Source: three-view drawing plus pictorial views. Frame: mm from the lowest corner of the part. A direction names the side the tool comes from. Round coordinates to 2 decimals unless told otherwise and drop trailing zeros. Write each loop counter-clockwise with the first axis right and the second up, starting at its lowest first coordinate (ties: lowest second). Pieces come first, ordered by that corner, then holes. Notation, with made-up numbers: M 8,-33.75 L 55,-33.75 A30 cw 55,-11.75 Z; hole C 23.5,60.25 d2. An arc over 180 degrees is marked long. Answer in a Markdown table with one row per item.
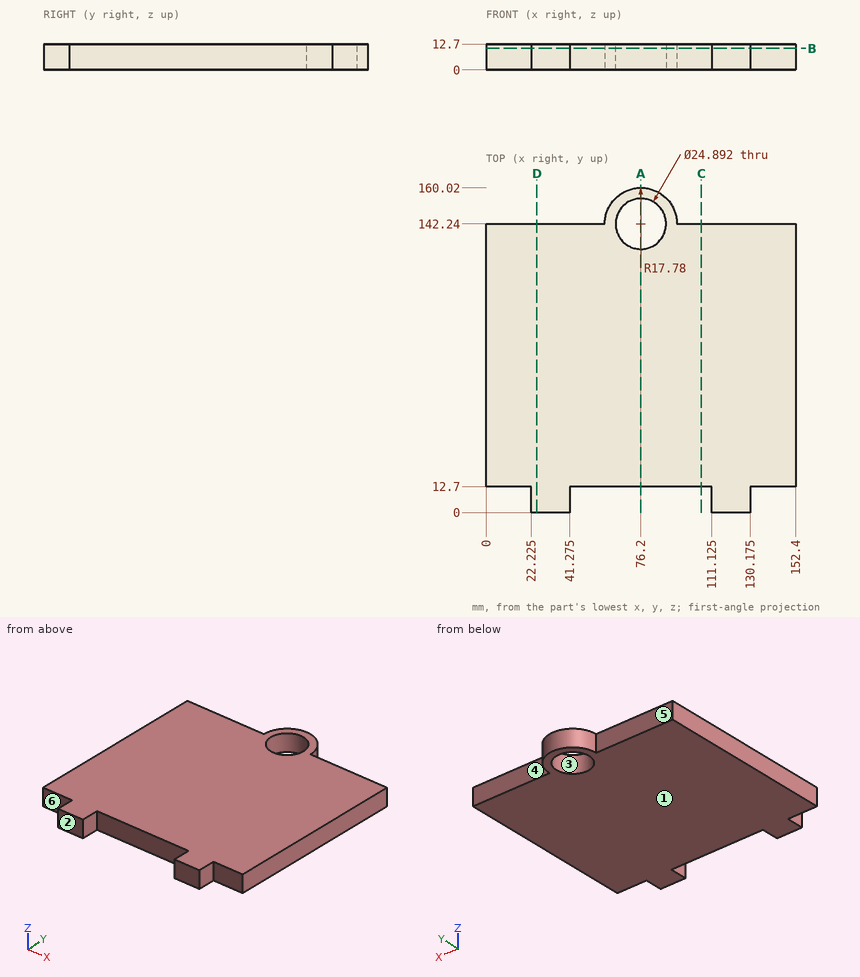
Q1. Section B-B (z = 10.5). Return loops of the section in (x, y) (3 decimals), and give its area (3 significant figures).
Solutions:
| item | result |
|---|---|
| outline | M 0,12.7 L 22.225,12.7 L 22.225,0 L 41.275,0 L 41.275,12.7 L 111.125,12.7 L 111.125,0 L 130.175,0 L 130.175,12.7 L 152.4,12.7 L 152.4,142.24 L 93.98,142.24 A17.78 ccw 58.42,142.24 L 0,142.24 Z; hole C 76.2,142.24 d24.892 |
| area | 20,200 mm2 |
Q2. Contact query for flat-ended pins moving along their axis: pin 1 Ø2 at (x, z) = (47, 6.5) entering from +Y; pin 2 Ø4 at (y, z) = (5, 4) entering from +X (3 decimals); pin 3 Ø6.5 at (y, z) = (8.5, 4.5) entering from -X (3 decimals). Output: stop coordinate, or through.
Solutions:
| item | result |
|---|---|
| pin 1 | stops at y = 142.24 |
| pin 2 | stops at x = 130.175 |
| pin 3 | stops at x = 22.225 |
Q3. Pull-direction query (Y, two-part tool) for the marked faces 1, 2 and 3; classes: pulls with the +Y half, pulls with the -Y half, needs draft (parallel to the pull), parting line crosses it, or undercut.
Solutions:
| item | result |
|---|---|
| face 1 | needs draft |
| face 2 | pulls with the -Y half |
| face 3 | undercut |
Q4. Access query for the marked faces 4, 5 and 6. Directions: +Z, -Z, +X, -X, +Y, -Y. A direction counts if a zero-diameter tool reaches every point of the face in a straight line with its end or side. Return the directions, or none.
Solutions:
| item | result |
|---|---|
| face 4 | +Z, -Z, +X, +Y |
| face 5 | +Z, -Z, -X, +Y |
| face 6 | +Z, -Z, -X, -Y |
Q5. Section D-D (x = 25). Return loops of the section in (y, z).
Solutions:
| item | result |
|---|---|
| outline | M 0,0 L 142.24,0 L 142.24,12.7 L 0,12.7 Z |
Q6. Section A-A (x = 76.2). Return loops of the section in (y, z), and give its area (3 significant figures).
Solutions:
| item | result |
|---|---|
| outline | M 12.7,0 L 129.79,0 L 129.79,12.7 L 12.7,12.7 Z; M 154.69,0 L 160.02,0 L 160.02,12.7 L 154.69,12.7 Z |
| area | 1,550 mm2 |
Q7. Material intervals for probe 1 along Y at (x, z) = (25, 9.25); probe 2 along Y at (x, z) = (108, 7); probe 3 along Y at (x, z) = (71, 5.5), sorted ascending.
Solutions:
| item | result |
|---|---|
| probe 1 | y = 0 to 142.24 |
| probe 2 | y = 12.7 to 142.24 |
| probe 3 | y = 12.7 to 130.93, 153.55 to 159.24 |
Q8. Section C-C (x = 106). Return loops of the section in (y, z), and give its area (3 significant figures).
Solutions:
| item | result |
|---|---|
| outline | M 12.7,0 L 142.24,0 L 142.24,12.7 L 12.7,12.7 Z |
| area | 1,650 mm2 |
